Here's how the part is built. I have some questions about the finished solid (model axes, mm). A direction names the side the tool comes from. Round coordinates to 2 decimals unless told otherwise and drop trailing zeros. Write each loop counter-clockwise with the first axis right and the second up, starting at its lowest first coordinate (ties: lowest second). Pieces come first, ordered by that corner, then holes. Notation, with made-up numbers: M -3.5,72 L 15.5,72 A19 ccw 15.5,95 Z; hole C 32.25,37 d5. An arc over 180 degrees is marked long. Write item = value, one per line. Start each with the question number.
(1) On a 3-axis mill with a long thin cutter (end or side, diameter ignored), from which of +Z, -Z, +X, -X, +Y, -Y can I reach the whole of each face in a straight line? I mean faces 4 (the flat face through (-11.2, 3.4, 0)), 5 (the flat face through (-9.2, 15.4, 1)), 6 (the flat face through (-9.23, -15.05, 14)), 7 (the flat face through (18, 0, 14)), 8 (the flat face through (8.7, -15.4, 14)). Say none if no direction works.
(2) If we mould it in two halves opening along X, with no side actions, what happens to faces 1 (the flat face through (15.212, 8.652, 7.409)), 2 (the flat face through (-19.207, 0, 7)), 3 (the conical face through (9.305, -5.274, 7.231))? For each: released by +X, released by -X, zero draft, split by the parting line, or undercut.
(3) I need wall thicknesses on line 1 along Z through (x, y) = (0, -14.45); line 2 along X through (y, z) = (0, 11.75). Which ranges of each line are inside material? Lowest first, please.
(4) I want a section at C-C (z = 10). List the corners of the cut face in (x, y) for me.
(5) I want a section at B-B (z = 3). List the corners of the cut face in (x, y) for me, and give its area (3 significant figures).
(6) Will these pins go through, and if not, where does the flat tip stop? pin 1 Ø1 at (y, z) = (2.5, 8) entering from -X; pin 2 Ø1.9 at (x, z) = (0, 7.5) entering from -Y; pin 3 Ø4 at (x, y) = (6, -7) entering from -Z.
Autodesk Inventor part; units mm, degrees
ref_plane "Plan de construction1" through (0, 0, 1) normal (0, 0, -1) x (-1, 0, 0)
ref_plane "YZ Plane" through (0, 0, 0) normal (1, 0, 0) x (0, 1, 0)
ref_plane "XZ Plane" through (0, 0, 0) normal (0, 1, 0) x (-1, 0, 0)
sketch "Esquisse1" plane through (0, 0, 0) normal (1, 0, 0) x (0, 1, 0)
  line L0 (0, 0) -> (0, 17.727)
  line L1 (8.25, 5) -> (8.25, 15)
  line L2 (8.25, 5) -> (11, 5)
  line L3 (11, 5) -> (11, 0)
  line L4 (17.5, 14) -> (17.5, 1)
  line L5 (16.5, 0) -> (11, 0)
  line L6 (8.25, 15) -> (16.5, 15)
  line L7 (16.5, 15) -> (17.5, 14)
  line L8 (17.5, 1) -> (16.5, 0)
  dimension "d1" = 16.5
  dimension "d2" = 22
  dimension "d3" = 35
  dimension "d4" = 5
  dimension "d71" = 1
  dimension "d72" = 1
  dimension "d77" = 1
  dimension "d78" = 1
  dimension "d82" = 15
revolve "Révolution1" add sketch "Esquisse1" angle 360 about axis through (0, 0, 0) along (0, 0, 1)
ref_plane "Plan de construction1" through (0, 0, 1) normal (0, 0, -1) x (-1, 0, 0)
sketch "Esquisse2" plane through (0, 0, 1) normal (0, 0, -1) x (-1, 0, 0)
  line L0 (10.1036, 17.5) -> (20.2073, 0)
  line L1 (20.2073, 0) -> (10.1036, -17.5)
  line L2 (10.1036, -17.5) -> (-10.1036, -17.5)
  line L3 (-10.1036, -17.5) -> (-20.2073, 0)
  line L4 (-20.2073, 0) -> (-10.1036, 17.5)
  line L5 (-10.1036, 17.5) -> (10.1036, 17.5)
  circle A0 centre (0, 0) radius 17.5
  arc A1 (-15.1554, 8.75) -> (15.1554, 8.75) centre (0, 0) ccw
extrude "Extrusion1" add sketch "Esquisse2" against normal blind 13 contours L0 A0 L5 | L0 L1 A0 | A0 L4 L5 | A0 L3 L4 | L1 L2 A0 | A0 L2 L3
chamfer "Chanfrein1" distance 0.5 angle 45 2 edges at (0, -11, 0) (0, -11, 5)
chamfer "Chanfrein2" distance 2 angle 45 6 edges at (10.1036, 17.5, 7.5) (20.2073, 0, 7.5) (10.1036, -17.5, 7.5) (-10.1036, -17.5, 7.5) (-20.2073, 0, 7.5) (-10.1036, 17.5, 7.5)
sketch "Esquisse3" plane through (-8.1036, -17.5, 1) normal (0, -1, 0) x (1, 0, 0)
  line L0 (0, 13) -> (16.2073, 13)
  line L1 (-8.3964, -1) -> (24.6036, -1)
  line L2 (0, 0) -> (0, 13)
  point P0 (8.1036, -1)
  point P1 (8.1036, 6.5)
  point P2 (8.1036, 0)
  point P3 (16.2073, 0)
  point P4 (8.1036, 0)
  point P5 (8.1036, 13)
  point P6 (0, 6.5)
hole "Perçage1" at (0, -17.5, 7.5) direction (0, 1, 0) diameter 3.242 depth 6 tip angle 118
chamfer "Chanfrein4" distance 0.5 angle 45 2 edges at (0, -8.25, 15) (0, -8.25, 5)
chamfer "Chanfrein5" distance 1 angle 45 6 edges at (9.6036, 16.634, 14) (19.2073, 0, 14) (9.6036, -16.634, 14) (-9.6036, -16.634, 14) (-19.2073, 0, 14) (-9.6036, 16.634, 14)
pattern_circular "Réseau circulaire2" count 3 over 120 about axis through (0, 0, -10) along (0, 0, 1) of "Perçage1" both ways yes
equation "\"d72\" = d71"
equation "\"d78\" = d77"
properties part number "support_canon" material "Aluminium 6061"
Returned:
q1.face_4 = -Z, +X, -X, +Y, -Y
q1.face_5 = -Z, -X, +Y
q1.face_6 = +Z, -X, -Y
q1.face_7 = +Z, +X
q1.face_8 = +Z, +X, -Y
q2.face_1 = released by +X
q2.face_2 = released by -X
q2.face_3 = undercut
q3.line_1 = 0 to 5.88, 9.12 to 15
q3.line_2 = -19.21 to -8.25, 8.25 to 19.21
q4.outline = M -19.21,-1.73 L -11.1,-15.77 L -8.1,-17.5 L 8.1,-17.5 L 11.1,-15.77 L 19.21,-1.73 L 19.21,1.73 L 11.1,15.77 L 8.1,17.5 L -8.1,17.5 L -11.1,15.77 L -19.21,1.73 Z; hole C 0,0 d16.5
q5.outline = M -19.21,-1.73 L -11.1,-15.77 L -8.1,-17.5 L 8.1,-17.5 L 11.1,-15.77 L 19.21,-1.73 L 19.21,1.73 L 11.1,15.77 L 8.1,17.5 L -8.1,17.5 L -11.1,15.77 L -19.21,1.73 Z; hole C 0,0 d22
q5.area = 670 mm²
q6.pin_1 = -19.05
q6.pin_2 = -11.1
q6.pin_3 = 0.28
